Source: CAD feature listing. Evaluate the final solid. Frame: model axes, mm. Face numbers are marked on the shaded views. A direction names the side the tool comes from. Coordinates: 2 decimals unless noted, no trailing zeros. Loops run counter-clockwise (first coordinate to the right, second up) from the corner with the lowest first, then second, coordinate; pieces in that order, holes last. Notation, with made-up numbers: (33, 57.5) - (79, 57.5) arc R19 cw to (79, 92.5) - close; hole circle Ø6 at (8, 49.25). An arc over 180 degrees is marked (long way). Use one line per item in the form item = value. Start each with the question number.
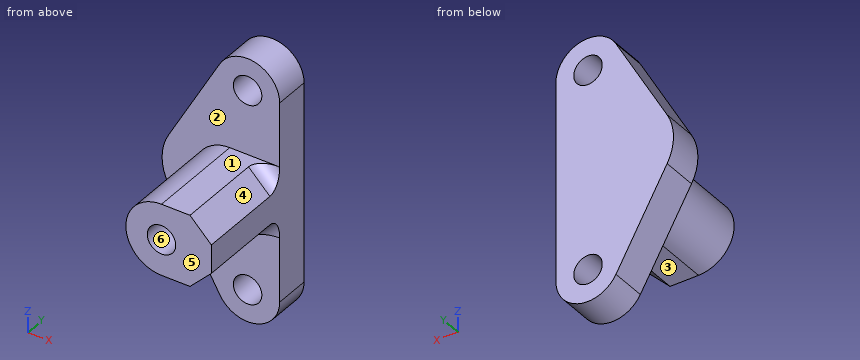
Autodesk Inventor part; units mm, degrees
ref_plane "YZ Plane" through (0, 0, 0) normal (1, 0, 0) x (0, 1, 0)
ref_plane "XZ Plane" through (0, 0, 0) normal (0, 1, 0) x (-1, 0, 0)
ref_plane "XY Plane" through (0, 0, 0) normal (0, 0, 1) x (1, 0, 0)
sketch "Sketch1" plane through (0, 0, 0) normal (0, 1, 0) x (-1, 0, 0)
  circle A0 centre (0, 0) radius 2.5
  dimension "d0" = 5
extrude "Extrusion1" add sketch "Sketch1" along normal blind 7
sketch "Sketch2" plane through (0, 7, 0) normal (0, 1, 0) x (1, 0, 0)
  circle A0 centre (0, 0) radius 2.5
  circle A1 centre (0, 0) radius 3.5
  line L0 (0, 0) -> (2.5, 0)
  line L1 (2.5, 0) -> (2.5, 7)
  line L2 (2.5, 0) -> (2.5, -7)
  circle A2 centre (2.5, -7) radius 2.25
  circle A3 centre (2.5, 7) radius 2.25
  line L3 (0, 0) -> (-3.0512, -1.7147)
  line L4 (-3.0512, -1.7147) -> (0.5385, -8.1023)
  line L5 (2.5, -7) -> (0.5385, -8.1023)
  line L6 (2.5, 7) -> (0.5385, 8.1023)
  line L7 (0, 0) -> (-3.0512, 1.7147)
  line L8 (-3.0512, 1.7147) -> (0.5385, 8.1023)
  line L9 (2.5, -7) -> (4.75, -7)
  line L10 (2.5, 7) -> (4.75, 7)
  line L11 (4.75, 7) -> (4.75, -7)
  dimension "d3" = 7
  dimension "d4" = 2.5
  dimension "d5" = 7
  dimension "d6" = 7
  dimension "d7" = 4.5
  dimension "d8" = 4.5
extrude "Extrusion2" add sketch "Sketch2" along normal blind 3
sketch "Sketch4" plane through (0, 0, 0) normal (0, -1, 0) x (1, 0, 0)
  line L0 (4.75, 7) -> (4.75, -7)
  arc A0 (4.75, 7) -> (0.5385, 8.1023) centre (2.5, 7) ccw
  line L1 (-3.0512, 1.7147) -> (0.5385, 8.1023)
  arc A1 (-3.0512, 1.7147) -> (-3.0512, -1.7147) centre (0, 0) ccw
  line L2 (0.5385, -8.1023) -> (-3.0512, -1.7147)
  arc A2 (0.5385, -8.1023) -> (4.75, -7) centre (2.5, -7) ccw
  circle A3 centre (0, 0) radius 2.5
extrude "Extrusion4" add sketch "Sketch4" along normal blind 3 contours L0 A2 L2 A1 L1 A0 | A3
sketch "Sketch5" plane through (0, 7, 0) normal (0, -1, 0) x (1, 0, 0)
  circle A0 centre (0, 0) radius 2.5
  line L0 (4.75, -7) -> (4.75, 7)
  line L1 (0, 0) -> (0, 2.5)
  circle A1 centre (0, 0) radius 2.5
  line L2 (4.75, -7) -> (4.75, 7)
  line L3 (0, 2.5) -> (4.75, 2.5)
  line L4 (4.75, 2.5) -> (4.75, -2.5)
  line L5 (4.75, -2.5) -> (0, -2.5)
  line L6 (0, -2.5) -> (0, 2.5)
  point P0 (6.25, 2.5)
  point P1 (4.75, 7.3386)
  point P2 (4.75, 2.5)
extrude "Extrusion5" add sketch "Sketch5" along normal up to surface (7 mm away) contours A0 L3 L0 L5
sketch "Sketch7" plane through (0, -3, 0) normal (0, -1, 0) x (1, 0, 0)
  arc A0 (0.5385, -8.1023) -> (4.75, -7) centre (2.5, -7) ccw
  line L0 (4.75, -7) -> (4.75, 7)
  arc A1 (4.75, 7) -> (0.5385, 8.1023) centre (2.5, 7) ccw
  line L1 (0.5385, 8.1023) -> (-3.0512, 1.7147)
  arc A2 (-3.0512, 1.7147) -> (-3.0512, -1.7147) centre (0, 0) ccw
  line L2 (-3.0512, -1.7147) -> (0.5385, -8.1023)
  circle A3 centre (2.5, -7) radius 1
  circle A4 centre (2.5, 7) radius 1
  dimension "d27" = 2
  dimension "d28" = 2
extrude "Extrusion7" cut sketch "Sketch7" against normal up to surface (13 mm away) contours A3 | A4
thicken "Thicken1" operation add thickness 0.5 both sides no extend neighbours yes toward (0, 1, 0) faces at (0.73, -3, -0.5716)
thicken "Thicken2" operation add thickness 0.5 both sides no extend neighbours yes toward (0, -1, 0) faces at (0.73, 10, 0.5716)
sketch "Sketch8" plane through (0, 0, 0) normal (0, 1, 0) x (1, 0, 0)
  arc A0 (0, 2.5) -> (0, -2.5) centre (0, 0) ccw
  line L0 (0, 0) -> (1.5, 0)
  circle A1 centre (1.5, 0) radius 2.5
  line L1 (0, 2.5) -> (4.75, 2.5)
  line L2 (4.75, -2.5) -> (0, -2.5)
  line L3 (1.5, 0) -> (1.5, 2.5)
  line L4 (1.5, 2.5) -> (0, 2.5)
  line L5 (1.5, 0) -> (1.375, -2.5)
  line L6 (1.375, -2.5) -> (0, -2.5)
  line L7 (0, -2.5) -> (1.5, -2.5)
  line L8 (1.5, -2.5) -> (1.5, 2.5)
  line L9 (1.5, 2.5) -> (0, 2.5)
  line L10 (0, 2.5) -> (0, -2.5)
  point P0 (2.75, 2.5)
  point P1 (2.75, -2.5)
  point P2 (1.3752, -2.4969)
  point P3 (3.75, 2.5)
  point P4 (3.75, -2.5)
  dimension "d36" = 5
  dimension "d35" = 1.5
extrude "Extrusion8" cut sketch "Sketch8" along normal up to surface (7 mm away) contours L10 A1 A0 | L1 A1 L10 | L10 A1 L5 L2
sketch "Sketch11" plane through (0, 7, 0) normal (0, -1, 0) x (1, 0, 0)
  circle A0 centre (2.5, 7) radius 1
  circle A1 centre (2.5, -7) radius 1
  line L0 (-3.0512, 1.7147) -> (0.5385, 8.1023)
  arc A2 (4.75, 7) -> (0.5385, 8.1023) centre (2.5, 7) ccw
  line L1 (4.75, 7) -> (4.75, -7)
  arc A3 (0.5385, -8.1023) -> (4.75, -7) centre (2.5, -7) ccw
  line L2 (0.5385, -8.1023) -> (-3.0512, -1.7147)
  arc A4 (-3.0512, 1.7147) -> (-3.0512, -1.7147) centre (0, 0) ccw
extrude "Extrusion9" cut sketch "Sketch11" along normal up to surface (7 mm away)
sketch "Sketch12" plane through (0, 0, 0) normal (0, 1, 0) x (1, 0, 0)
  circle A0 centre (2.5, -7) radius 1
  circle A1 centre (2.5, 7) radius 1
  line L0 (4.75, 7) -> (4.75, -7)
  arc A2 (4.75, 7) -> (0.5385, 8.1023) centre (2.5, 7) ccw
  line L1 (-3.0512, 1.7147) -> (0.5385, 8.1023)
  arc A3 (-3.0512, 1.7147) -> (-3.0512, -1.7147) centre (0, 0) ccw
  line L2 (0.5385, -8.1023) -> (-3.0512, -1.7147)
  arc A4 (0.5385, -8.1023) -> (4.75, -7) centre (2.5, -7) ccw
  line L3 (4.75, 7) -> (4.75, -7)
  line L4 (4.75, 0) -> (3.75, 0)
  line L5 (3.75, 0) -> (1.25, 0)
  circle A5 centre (1.25, 0) radius 2.5
  line L6 (1.25, 0) -> (1.25, -2.5)
  line L7 (1.25, -2.5) -> (4.75, -2.5)
  line L8 (4.75, -2.5) -> (4.75, 2.5)
  line L9 (4.75, 2.5) -> (1.25, 2.5)
  line L10 (1.25, 2.5) -> (1.25, -2.5)
  point P0 (4.75, 2.5)
  dimension "d45" = 1
  dimension "d46" = 2.5
  dimension "d47" = 5
  dimension "d48" = 3.5
  dimension "d49" = 5
extrude "Extrusion10" add sketch "Sketch12" along normal up to surface (7 mm away) contours L0 L4 A5 L9 | L0 L7 A5 L4 | L10 L6 A5 | A5 L5 L10 | A5 L6 L5
chamfer "Chamfer2" distance 1.5 angle 45 2 edges at (4.75, 3.5, 2.5) (4.75, 3.5, -2.5)
sketch "Sketch13" plane through (0, 0, 0) normal (0, 1, 0) x (1, 0, 0)
  circle A0 centre (2.5, -7) radius 1
  circle A1 centre (2.5, 7) radius 1
  line L0 (-3.0512, 1.7147) -> (0.5385, 8.1023)
  arc A2 (4.75, 7) -> (0.5385, 8.1023) centre (2.5, 7) ccw
  line L1 (4.75, 7) -> (4.75, -7)
  arc A3 (0.5385, -8.1023) -> (4.75, -7) centre (2.5, -7) ccw
  line L2 (0.5385, -8.1023) -> (-3.0512, -1.7147)
  arc A4 (-3.0512, 1.7147) -> (-3.0512, -1.7147) centre (0, 0) ccw
extrude "Extrusion11" cut sketch "Sketch13" against normal blind 10
sketch "Sketch14" plane through (0, 0, 0) normal (0, -1, 0) x (1, 0, 0)
  line L0 (4.75, -1) -> (3.25, -2.5)
  line L1 (4.75, 1) -> (4.75, -1)
  line L2 (3.25, 2.5) -> (4.75, 1)
  line L3 (3.25, 2.5) -> (1.25, 2.5)
  arc A0 (1.25, 2.5) -> (1.25, -2.5) centre (1.25, 0) ccw
  line L4 (1.25, -2.5) -> (3.25, -2.5)
  circle A1 centre (1.25, 0) radius 1
  point P0 (0, 0)
  dimension "d58" = 2
extrude "Extrusion12" cut sketch "Sketch14" against normal blind 5 contours A1
fillet "Fillet3" radius 1 2 edges at (4, 7, -1.75) (4, 7, 1.75)
properties part number "belt_tendor_1"
(1) Contact query for flat-ended pins moving along their axis: pin 1 (0.6 mm diameter, centred on x = 1, z = 0.5, fed in from -Y); pin 2 (1 mm diameter, centred on x = 2.5, y = 2.5, fed in from +Z); pin 3 (3 mm diameter, centred on x = 1, y = 6.5, fed in from -Z); pin 4 (1.6 mm diameter, centred on x = 2.5, z = -7, fed in from +Y). Output: stop coordinate, or through.
(2) Access query for the marked faces 1, 2 and 3. Directions: +Z, -Z, +X, -X, +Y, -Y. A direction counts if a zero-diameter tool reaches every point of the face in a straight line with its end or side. Return the directions, or none.
(3) Material intervals for line 1 (Z direction, x = 2.5, y = 8.45); line 2 (Z direction, x = 1.25, y = 3.35); line 3 (Y direction, x = 1.25, z = -6), sorted ascending.
(4) Mould query, pull axis Z, two halves, no side actions, for the marked faces 4, 5 and 6. Classes: +Z half, -Z half, draft (parallel to the pull), parting line (faces both ways), or undercut.
(5) Cut plane C-C, the plane z = 0. Output: boundary loops of the cut face in (x, y), plus the area to 3 significant figures.
(6) Cut plane A-A, the plane y = 8. Output: boundary loops of the cut face in (x, z), plus the area to 3 significant figures.
(7) Cut plane B-B, the plane y = 2.5. Output: boundary loops of the cut face in (x, z), plus the area to 3 significant figures.
(8) Cut plane D-D, the plane x = -0.75. Output: boundary loops of the cut face in (y, z).
Recorded:
q1.pin_1 = 5
q1.pin_2 = 2.5
q1.pin_3 = -9.25
q1.pin_4 = through
q2.face_1 = +Z, +X, -X, -Y
q2.face_2 = -X, -Y
q2.face_3 = -Z, +X, -X, -Y
q3.line_1 = -9.25 to -8, -6 to 6, 8 to 9.25
q3.line_2 = -2.5 to -1, 1 to 2.5
q3.line_3 = 7 to 9.5
q4.face_4 = +Z half
q4.face_5 = draft
q4.face_6 = undercut
q5.outline = (-3.5, 7) - (-1.25, 7) - (-1.25, 0) - (0.25, 0) - (0.25, 5) - (2.25, 5) - (2.25, 0) - (4.75, 0) - (4.75, 9.5) - (-3.5, 9.5) - close
q5.area = 52.6 mm²
q6.outline = (-3.05, -1.71) - (0.54, -8.1) arc R2.25 ccw to (4.75, -7) - (4.75, 7) arc R2.25 ccw to (0.54, 8.1) - (-3.05, 1.71) arc R3.5 ccw to start; hole circle Ø2 at (2.5, -7); hole circle Ø2 at (2.5, 7)
q6.area = 104 mm²
q7.outline = (1.25, -2.5) - (3.25, -2.5) - (4.75, -1) - (4.75, 1) - (3.25, 2.5) - (1.25, 2.5) arc R2.5 ccw to start; hole circle Ø2 at (1.25, 0)
q7.area = 21.9 mm²
q8.outline = (0, -1.5) - (7, -1.5) - (7, -5.81) - (9.5, -5.81) - (9.5, 5.81) - (7, 5.81) - (7, 1.5) - (0, 1.5) - close
